Autodesk Inventor part; units mm, degrees
ref_plane "YZ Plane" through (0, 0, 0) normal (1, 0, 0) x (0, 1, 0)
ref_plane "XZ Plane" through (0, 0, 0) normal (0, 1, 0) x (-1, 0, 0)
ref_plane "XY Plane" through (0, 0, 0) normal (0, 0, 1) x (1, 0, 0)
sketch "Sketch1" plane through (0, 0, 0) normal (0, 1, 0) x (-1, 0, 0)
  line L0 (-85.725, 9.525) -> (85.725, 9.525)
  line L1 (85.725, 9.525) -> (85.725, -9.525)
  line L2 (85.725, -9.525) -> (-85.725, -9.525)
  line L3 (-85.725, -9.525) -> (-85.725, 9.525)
  line L4 (-85.725, 9.525) -> (85.725, -9.525) construction
  line L5 (85.725, 9.525) -> (-85.725, -9.525) construction
  point P0 (0, 0)
  dimension "d0" = 171.45
  dimension "d1" = 19.05
extrude "Extrusion1" add sketch "Sketch1" along normal blind 12.7
sketch "Sketch2" plane through (85.725, 0, 9.525) normal (1, 0, 0) x (0, 0, -1)
  line L0 (0, 0) -> (0, 12.7)
  line L1 (0, 6.35) -> (19.05, 6.35)
  line L2 (19.05, 0) -> (19.05, 12.7)
  circle A0 centre (9.525, 6.35) radius 2.3812
  point P0 (9.525, 0)
  dimension "d4" = 4.7625
extrude "Extrusion2" cut sketch "Sketch2" against normal blind 12.7
sketch "Sketch3" plane through (-85.725, 0, 9.525) normal (0, 0, 1) x (1, 0, 0)
  line L0 (0, 0) -> (0, 12.7)
  line L1 (0, 6.35) -> (9.525, 6.35)
  circle A0 centre (9.525, 6.35) radius 2.3812
  point P0 (85.725, 0)
  dimension "d7" = 9.525
  dimension "d8" = 4.7625
extrude "Extrusion3" cut sketch "Sketch3" against normal blind 12.7
properties part number "shootFrame" material "Wood (Birch)"
Geometry: final body of the model. Coordinates: model frame, mm. A direction names the side the tool comes from. Give positions to 0.01 mm unless a question says otherwise; leave off trailing zeros. Loops run counter-clockwise (first coordinate to the right, second up) from the corner with the lowest first, then second, coordinate; pieces in that order, holes last. Notation, with made-up numbers: (61, 76) -> (106, 76) arc R30 ccw to (106, 114) -> close; hole circle Ø4 at (3.25, 19.5). An arc over 180 degrees is marked (long way). Use one line per item in the form item = value.
Item 1: Section query B-B on y = 6.35. Output: boundary loops of the cut face in (x, z) (3 decimals), and give its area (3 significant figures).
A:
outline = (-85.725, -9.525) -> (85.725, -9.525) -> (85.725, -2.381) -> (73.025, -2.381) -> (73.025, 2.381) -> (85.725, 2.381) -> (85.725, 9.525) -> (-73.819, 9.525) -> (-73.819, -3.175) -> (-78.581, -3.175) -> (-78.581, 9.525) -> (-85.725, 9.525) -> close
area = 3,150 mm^2
Item 2: Draft query along Z for faces 1 (the face through (73.025, 6, 0)), 2 (the face through (-76, 6, -3.175)), 3 (the face through (-85.725, 6, 0)). Return one class per face: pulls with the +Z half, pulls with the -Z half, needs draft (parallel to the pull), parting line crosses it, or undercut.
A:
face_1 = undercut
face_2 = pulls with the +Z half
face_3 = needs draft
Item 3: Access query for faces 4 (the face through (1, 12.7, 0)), 5 (the face through (79.46, 7.07, -2.27)), 6 (the face through (-78.58, 6.45, 3.26)). Directions: +Z, -Z, +X, -X, +Y, -Y. A direction counts if a zero-diameter tool reaches every point of the face in a straight line with its end or side. Return the directions, or none.
A:
face_4 = +Z, -Z, +X, -X, +Y
face_5 = +X
face_6 = +Z
Item 4: Line query: probe 1 along Y at (x, z) = (-76.2, 6.5); probe 2 along Z at (x, y) = (82.5, 6.35) (3 decimals); probe 3 along X at (y, z) = (6.35, 4) (3 decimals). Output: solid intervals per line, ascending.
A:
probe_1 = 0 to 3.97, 8.73 to 12.7
probe_2 = -9.525 to -2.381, 2.381 to 9.525
probe_3 = -85.725 to -78.581, -73.819 to 85.725
Item 5: Pin query (flat end, axial travel): P1, Ø3, axis at y = 6.35, z = 0, coming from the +X side (3 decimals). Return the tip coordinate at first contact, or that it passes through.
A:
P1 = 73.025
Item 6: Section query C-C on x = -76.2. Output: boundary loops of the cut face in (y, z) (3 decimals).
A:
outline = (0, -9.525) -> (12.7, -9.525) -> (12.7, 9.525) -> (8.731, 9.525) -> (8.731, -3.175) -> (3.969, -3.175) -> (3.969, 9.525) -> (0, 9.525) -> close
Item 7: Section query A-A on z = 0. Output: boundary loops of the cut face in (x, y) (3 decimals), and give its area (3 significant figures).
A:
outline = (-85.725, 0) -> (85.725, 0) -> (85.725, 3.969) -> (73.025, 3.969) -> (73.025, 8.731) -> (85.725, 8.731) -> (85.725, 12.7) -> (-85.725, 12.7) -> close; hole circle Ø4.762 at (-76.2, 6.35)
area = 2,100 mm^2
